Can you work these out from the model? Positions are in its coordinate system, mm. A direction names the side the tool comes from. Coordinates: 2 decimals unless noted, no trailing zeros. Order: outer loops, then holes, each group sorted by start corner. A loop starts at its lowest first (then second) coordinate and runs counter-clockwise, first axis right, second up. Notation, with made-up numbers: (67.5, 5) - (120.5, 5) arc R18 ccw to (120.5, 32) - close; hole circle Ø8 at (83, 50). An arc over 180 degrees is marked (long way). Use a Markdown table: item, result. Add a question column.
(1) I want a section at A-A (x = 19.05). State how many separate pieces and enclosed holes the cut face has, and give its area (3 significant figures).
(2) On a 3-axis mill with a long thin cutter (end or side, diameter ignored), from which of +Z, -Z, +X, -X, +Y, -Y can I reach the whole of each face in a straight line? I mean faces 1 (the flat face through (36.512, 150, -6)), 2 (the flat face through (19.1, 303.7, -11.6)). Say none if no direction works.
(3) We'd pull the mould along Z, two halves only. Please class faces 3 (the flat face through (3, 150, -1.587)), 4 (the flat face through (4, 150, -12.7)), 5 (the flat face through (19.1, 1.1, -11.6)): pulls with the +Z half, pulls with the -Z half, needs draft (parallel to the pull), parting line crosses it, or undercut.
(4) For pin 1 Ø5.5 at (x, y) = (19.05, 196.85) entering from -Z, with a flat end and sliding along its axis, tell me the tip position at first contact or that it passes through.
(5) I want a section at B-B (y = 196.85). List the corners of the cut face in (x, z) for me (1 decimal).
(6) If I drill on L1, parallel to Z at x = 35, y = 280; L2, parallel to X at y = 181, z = -7; L3, parallel to Y at x = 19.05, z = -12.3 (3 decimals), over which ranges is the centre line in solid material (lowest first)? Write a range as [from, to].
(7) I want a section at C-C (y = 284). List the corners of the cut face in (x, z) for me (1 decimal), and give its area (3 significant figures).
```python
from build123d import *

# Parameters (mm, degrees)
SKETCH1_W           = 34.925
SKETCH1_H           = 9.525
BOSS_EXTRUDE1_DEPTH = 304.8
SKETCH2_R           = 12.7
SKETCH2_R_2         = 3.175
CUT_EXTRUDE1_DEPTH  = 13.7
CUT_EXTRUDE2_DEPTH  = 39.1


with BuildPart() as part:
    # Sketch1 → Boss-Extrude1 (new body)
    with BuildSketch(Plane(origin=(0, 0, 0), x_dir=(1, 0, 0), z_dir=(0, 1, 0))):
        with BuildLine():
            Line((1.5875, 0), (36.5125, 0))
            ThreePointArc((36.5125, 0), (37.635032015, 0.464967985), (38.1, 1.5875))
            Line((38.1, 1.5875), (38.1, 11.1125))
            ThreePointArc((38.1, 11.1125), (37.635032015, 12.235032015), (36.5125, 12.7))
            Line((36.5125, 12.7), (1.5875, 12.7))
            ThreePointArc((1.5875, 12.7), (0.464967985, 12.235032015), (0, 11.1125))
            Line((0, 11.1125), (0, 1.5875))
            ThreePointArc((0, 1.5875), (0.464967985, 0.464967985), (1.5875, 0))
        make_face()
        with Locations((19.05, 6.35)):
            Rectangle(SKETCH1_W, SKETCH1_H, mode=Mode.SUBTRACT)
    extrude(amount=BOSS_EXTRUDE1_DEPTH)

    # Sketch2 → Cut-Extrude1 (cut, through all)
    with BuildSketch(Plane.XY):
        with Locations((19.05, 152.4)):
            Circle(SKETCH2_R)
        with Locations((19.05, 196.85)):
            Circle(SKETCH2_R_2)
        with Locations((19.05, 234.95)):
            Circle(SKETCH2_R)
    extrude(amount=-CUT_EXTRUDE1_DEPTH, mode=Mode.SUBTRACT)

    # Sketch3 → Cut-Extrude2 (cut, through all)
    with BuildSketch(Plane(origin=(38.1, 0, 0), x_dir=(0, 0, -1), z_dir=(1, 0, 0))):
        Polygon((0, 0), (12.7, 0), (0, 12.7), align=None)
        Polygon((0, 304.8), (12.7, 304.8), (0, 292.1), align=None)
    extrude(amount=-CUT_EXTRUDE2_DEPTH, mode=Mode.SUBTRACT)


solid = part.part
```
Answers follow:
| question | item | result |
|---|---|---|
| 1 | separate pieces | 8 |
| 1 | enclosed holes | 0 |
| 1 | area | 746 mm² |
| 2 | face 1 | +Y, -Y |
| 2 | face 2 | +Z, +X, -X, +Y |
| 3 | face 3 | undercut |
| 3 | face 4 | pulls with the -Z half |
| 3 | face 5 | pulls with the +Z half |
| 4 | pin 1 | passes through |
| 5 | outline | (0, -11.1) arc R1.6 ccw to (1.6, -12.7) - (15.9, -12.7) - (15.9, -11.1) - (1.6, -11.1) - (1.6, -1.6) - (15.9, -1.6) - (15.9, 0) - (1.6, 0) arc R1.6 ccw to (0, -1.6) - close; (22.2, -12.7) - (36.5, -12.7) arc R1.6 ccw to (38.1, -11.1) - (38.1, -1.6) arc R1.6 ccw to (36.5, 0) - (22.2, 0) - (22.2, -1.6) - (36.5, -1.6) - (36.5, -11.1) - (22.2, -11.1) - close |
| 6 | L1 | z = [-12.7, -11.11], [-1.59, 0] |
| 6 | L2 | x = [0, 1.59], [36.51, 38.1] |
| 6 | L3 | y = [0.4, 139.7], [165.1, 193.675], [200.025, 222.25], [247.65, 304.4] |
| 7 | outline | (0, -11.1) arc R1.6 ccw to (1.6, -12.7) - (36.5, -12.7) arc R1.6 ccw to (38.1, -11.1) - (38.1, -1.6) arc R1.6 ccw to (36.5, 0) - (1.6, 0) arc R1.6 ccw to (0, -1.6) - close; hole (1.6, -11.1) - (36.5, -11.1) - (36.5, -1.6) - (1.6, -1.6) - close |
| 7 | area | 149 mm² |
